Answer from the drawing. Dimensions are ordinates in mm from the lowest x, y and z of the part. A direction names the side the tool comes from. Round coordinates to 2 decimals unless told otherwise and drop trailing zeros. Write each loop counter-clockwise with the first axis right and the second up, starting at its lowest first coordinate (ties: lowest second). Pieces come first, ordered by that corner, then holes. Notation, with made-up numbers: (61, -32.75) - (76, -32.75) arc R30 cw to (76, 0.25) - close; hole circle Ø6 at (64.25, 44.25). An arc over 180 degrees is marked (long way). One line per item, written item: value. Start each with the question number.
(1) Flat-ended cylindrical pins translate along their axes: pin 1 Ø1 at (y, z) = (6, 8) entering from -X; pin 2 Ø1.8 at (x, y) = (14.5, 6.5) entering from +Z; pin 3 Ø1 at (x, z) = (9.5, 2) entering from -Y. Find the tip coordinate at first contact, or state that the pin passes through.
(2) A cutting plane is placed at A-A, the plane x = 6.25. Determine the outline of the cut face in (y, z), plus the area to 3 significant figures.
(3) For the marked faces 1 and 2, determine the directions among +Z, -Z, +X, -X, +Y, -Y from which every point of the face is accessible in a straight line to the end or side of a thin tool.
(4) Find the intervals of material crossed by L1, parallel to X at y = 1.45, z = 5; L2, parallel to Y at x = 14.25, z = 11.75; L3, parallel to Z at x = 2.75, y = 8.75, in increasing order.
(5) A cutting plane is placed at B-B, the plane z = 2.25. Determine the outline of the cut face in (x, y).
(6) A cutting plane is placed at D-D, the plane y = 1.5. Determine the outline of the cut face in (x, z), plus the area to 3 significant figures.
(7) The mould has two halves that part along Y. Classify the marked faces 3, 4 and 5: +Y half, -Y half, draft (parallel to the pull), parting line (faces both ways), or undercut.
(8) A cutting plane is placed at C-C, the plane x = 10. Determine the outline of the cut face in (y, z), plus the area to 3 significant figures.
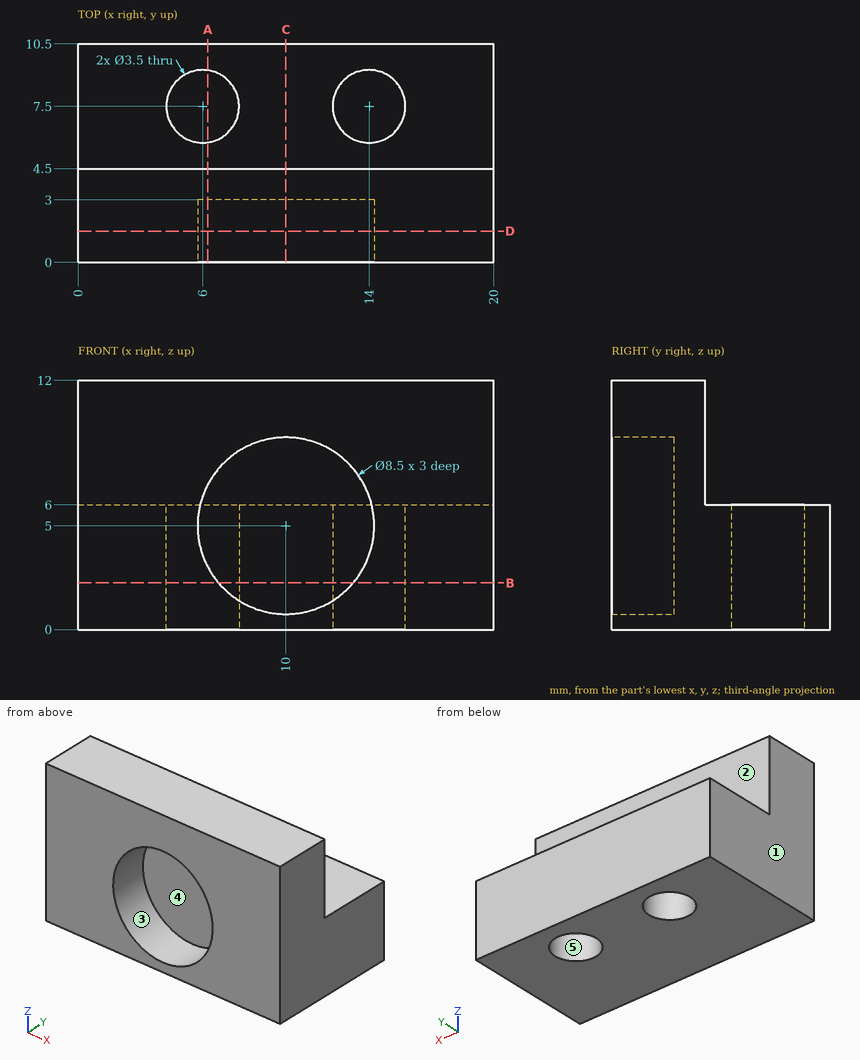
Here are the results:
1. pin 1: through
1. pin 2: z = 6
1. pin 3: y = 3
2. outline: (0, 0) - (5.77, 0) - (5.77, 6) - (4.5, 6) - (4.5, 12) - (0, 12) - (0, 7) - (3, 7) - (3, 3) - (0, 3) - close; (9.23, 0) - (10.5, 0) - (10.5, 6) - (9.23, 6) - close
2. area: 57.2 mm²
3. face 1: +Z, -Z, -X, +Y, -Y
3. face 2: +Z, +X, -X, +Y
4. L1: 0 to 5.75, 14.25 to 20
4. L2: 0 to 4.5
4. L3: 0 to 6
5. outline: (0, 0) - (6.76, 0) - (6.76, 3) - (13.24, 3) - (13.24, 0) - (20, 0) - (20, 10.5) - (0, 10.5) - close; hole circle Ø3.5 at (6, 7.5); hole circle Ø3.5 at (14, 7.5)
6. outline: (0, 0) - (20, 0) - (20, 12) - (0, 12) - close; hole circle Ø8.5 at (10, 5)
6. area: 183 mm²
7. face 3: draft
7. face 4: -Y half
7. face 5: undercut
8. outline: (0, 0) - (10.5, 0) - (10.5, 6) - (4.5, 6) - (4.5, 12) - (0, 12) - (0, 9.25) - (3, 9.25) - (3, 0.75) - (0, 0.75) - close
8. area: 64.5 mm²
